Can you work these out from the model? Positions are in its coordinate system, mm. Coordinates: 2 decimals unless noted, no trailing zeros. Order: outer loops, then holes, each group sorted by start corner. A loop starts at its lowest first (then second) coordinate and runs counter-clockwise, first axis right, second up. Notation, with made-up numbers: (38.5, 78) -> (87.5, 78) arc R9 cw to (87.5, 91) -> close; hole circle Ø2 at (35.25, 47). An arc over 180 degrees is marked (long way). Write item = value, one per line.
```python
from build123d import *

# Parameters (mm, degrees)
EXTRUDE_1_DEPTH    = 160
CHAMFER1_SIZE      = 5
CHAMFER1_SIZE2     = 4.986026333
SKETCH1_R          = 2
CUT_EXTRUDE1_DEPTH = 5
LPATTERN1_COUNT    = 3
LPATTERN1_PITCH    = 40


with BuildPart() as part:
    # 草圖1 → 填料-伸長1 (new body)
    with BuildSketch(Plane.XY):
        Polygon((203.623972775, 1001.176903993), (198.623972775, 1001.176903993), (198.623972775, 1041.176903993), (203.623972775, 1041.162871417), align=None)
    extrude(amount=EXTRUDE_1_DEPTH)

    # Chamfer1
    chamfer1_edges = [part.edges().sort_by_distance(p)[0] for p in [
        (198.623972775, 1041.176903993, 80),
    ]]
    chamfer1_side = [part.faces().sort_by_distance(p)[0] for p in [
        (198.623972775, 1021.176903993, 80),
    ]]
    chamfer(chamfer1_edges, length=CHAMFER1_SIZE, length2=CHAMFER1_SIZE2, reference=chamfer1_side[0])

    # Sketch1 → Cut-Extrude1 (cut)
    with BuildSketch(Plane(origin=(203.623972775, 0, 0), x_dir=(0, 0, -1), z_dir=(1, 0, 0))):
        with Locations((-40, 1016.176903993)):
            Circle(SKETCH1_R)
    cut_extrude1 = extrude(amount=-CUT_EXTRUDE1_DEPTH, mode=Mode.SUBTRACT)

    # LPattern1: Cut-Extrude1 ×3
    with Locations(*[(0, 0, i * LPATTERN1_PITCH) for i in range(1, LPATTERN1_COUNT)]):
        add(cut_extrude1, mode=Mode.SUBTRACT)


solid = part.part
```
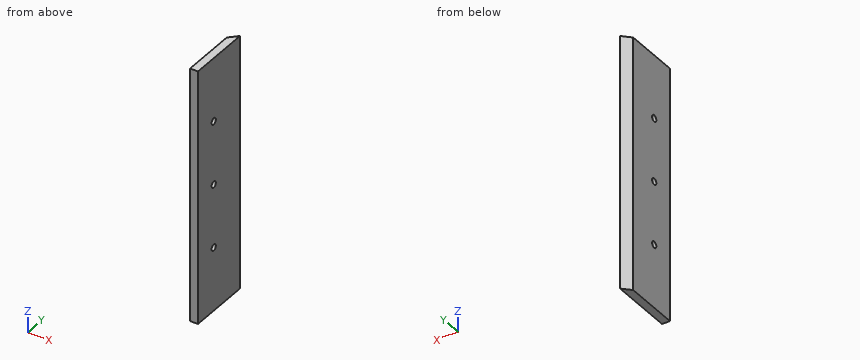
Item 1: I want a section at B-B, the plane x = 200.2. Please give me the cut outline in (y, z), plus the area to 3 significant figures.
A:
outline = (1001.18, 0) -> (1037.75, 0) -> (1037.75, 160) -> (1001.18, 160) -> close; hole circle Ø4 at (1016.18, 40); hole circle Ø4 at (1016.18, 80); hole circle Ø4 at (1016.18, 120)
area = 5,810 mm2
Item 2: I'm going to push a flat-ended pin straight in: P1, Ø3.5, axis at y = 1016.18, z = 80, coming from the -X side. Where does the tip first touch, or does it pass through?
A:
P1 = through
Item 3: If I drill on probe 1 along Z at (x, y) = (201.2, 1015.5); probe 2 along Y at (x, z) = (199.7, 40); probe 3 along Y at (x, z) = (201.5, 40), over which ranges is the centre line in solid material (lowest first)?
A:
probe_1 = 0 to 38.12, 41.88 to 78.12, 81.88 to 118.12, 121.88 to 160
probe_2 = 1001.18 to 1014.18, 1018.18 to 1037.25
probe_3 = 1001.18 to 1014.18, 1018.18 to 1039.05
